```python
from build123d import *

# Parameters (mm, degrees)
F1_DEPTH = 95.25
F2_W     = 101.5999999233
F2_H     = 31.75
F3_DEPTH = 63.5
F5_START = -63.5
F4_W     = 63.5
F4_H     = 127
F5_DEPTH = 127
F7_DEPTH = 63.5


with BuildPart() as f1:
    # F0 (on Front) → F1 (new body, symmetric)
    with BuildSketch(Plane.XZ):
        Polygon((0, 63.5), (0, 0), (95.25, 0), (95.25, 31.75), (158.75, 31.75), (158.75, 0), (254, 0), (254, 31.75), (317.5, 31.75), (317.5, 63.5), align=None)
    extrude(amount=F1_DEPTH, both=True)

    # F2 (on face) → F3 (join, symmetric)
    with BuildSketch(Plane.YZ.offset(254)):
        with Locations((44.4500000384, 15.875)):
            Rectangle(F2_W, F2_H)
    extrude(amount=F3_DEPTH, both=True)

    # F4 (on face) → F5 (join)
    with BuildSketch(Plane.XZ.offset(95.25).offset(F5_START)):
        with Locations((31.75, 127)):
            Rectangle(F4_W, F4_H)
    extrude(amount=-F5_DEPTH)

    # F6 (on face) → F7 (join)
    with BuildSketch(Plane.XY.offset(63.5)):
        Polygon((63.5, 95.25), (63.5, -6.35), (127, -6.35), (127, 57.15), (190.5, 57.15), (190.5, -6.35), (254, 69.85), (254, 95.25), align=None)
    extrude(amount=F7_DEPTH)


solid = f1.part
```
For this review, take the finished solid that the model builds, in its own axes (mm). A direction names the side the tool comes from. Give positions to 0.01 mm unless a question says otherwise; leave off trailing zeros. Order: outer loops, then holes, each group sorted by start corner. A loop starts at its lowest first (then second) coordinate and runs counter-clockwise, first axis right, second up.
1) The part is to be moulded in two halves that separate along X. For faces 1 (the face through (157, -95.25, 39)), 2 (the face through (0, 20, 94)), 3 (the face through (221.81, 31.22, 94.81)), 4 (the face through (127, -1, 31.75)), say which applies: released by +X, released by -X, zero draft, split by the parting line, or undercut.
2) Wall thickness on line 1 (X direction, y = 72, z = 147.5); line 2 (Z direction, x = 122, y = -7); line 3 (Z direction, x = 109.5, y = 10): over which ranges is each line inside the solid? List them lowest first.
3) For faces 5 (the face through (95.25, -1, 16)), 6 (the face through (190.5, 26, 95)), 7 (the face through (31, -31.75, 128)), 8 (the face through (95, -6.35, 95)), list the 3-axis set-ups (+Z, -Z, +X, -X, +Y, -Y) from which the entire face can be reached by the end or side of a thin tool; tool diameter is ignored.
4) Take a section at D-D (x = 237). Give the boundary of the cut face in (y, z).
5) Take a section at B-B (x = 50). Give the boundary of the cut face in (y, z).
6) Insertion check: pin 1 (19 mm diameter, centred on x = 140.5, y = -20, fed in from -Z); pin 2 (20.5 mm diameter, centred on y = 85.5, z = 89, fed in from +X); pin 3 (3 mm diameter, centred on y = 70.5, z = 134, fed in from +X). Each pin has a flat end and moves straight along its axis. Give the tip position at first contact, or say it passes through.
7) Take a section at C-C (z = 68). Give the boundary of the cut face in (x, y), then the cut area to 3 significant figures.
8) Take a section at A-A (y = 78). Give the boundary of the cut face in (x, z), then the cut area to 3 significant figures.
Derived:
1. face 1: zero draft
1. face 2: released by -X
1. face 3: released by +X
1. face 4: undercut
2. line 1: x = 0 to 63.5
2. line 2: z = 31.75 to 63.5
2. line 3: z = 31.75 to 127
3. face 5: -Z, +Y, -Y
3. face 6: +Z, -Y
3. face 7: +Z, +X, -X, -Y
3. face 8: +Z, +X, -Y
4. outline: (-95.25, 0) - (95.25, 0) - (95.25, 127) - (49.45, 127) - (49.45, 63.5) - (-95.25, 63.5) - close
5. outline: (-95.25, 0) - (95.25, 0) - (95.25, 190.5) - (-31.75, 190.5) - (-31.75, 63.5) - (-95.25, 63.5) - close
6. pin 1: stops at z = 31.75
6. pin 2: stops at x = 254
6. pin 3: stops at x = 63.5
7. outline: (0, -31.75) - (63.5, -31.75) - (63.5, -6.35) - (127, -6.35) - (127, 57.15) - (190.5, 57.15) - (190.5, -6.35) - (254, 69.85) - (254, 95.25) - (0, 95.25) - close
7. area: 21,000 mm2
8. outline: (0, 0) - (95.25, 0) - (95.25, 31.75) - (158.75, 31.75) - (158.75, 0) - (317.5, 0) - (317.5, 63.5) - (254, 63.5) - (254, 127) - (63.5, 127) - (63.5, 190.5) - (0, 190.5) - close
8. area: 38,300 mm2
